Geometry: final body of the model. Coordinates: model frame, mm. Give positions to 0.01 mm unless a question says otherwise; leave off trailing zeros. Loops run counter-clockwise (first coordinate to the right, second up) from the corner with the lowest first, then second, coordinate; pieces in that order, holes last. Notation, with made-up numbers: (-39.75, 51.5) - (-23.75, 51.5) arc R17 ccw to (-23.75, 75.5) - close; hole circle Ø6 at (78, 69). An arc over 180 degrees is marked (long way). Answer in a Markdown table with one row per item.
from build123d import *

# Parameters (mm, degrees)
F0_W     = 155.681744
F0_H     = 103.419952
F1_DEPTH = 20
F2_ANGLE = -180
F3_R     = 5


with BuildPart() as f1:
    # F0 (on Top) → F1 (new body)
    with BuildSketch(Plane.XY):
        Rectangle(F0_W, F0_H)
        with BuildLine():
            ThreePointArc((0, 30.621955), (21.652992, 21.652992), (30.621955, 0))
            ThreePointArc((30.621955, 0), (21.652992, -21.652992), (0, -30.621955))
            ThreePointArc((0, -30.621955), (-30.621955, 0), (0, 30.621955))
        make_face(mode=Mode.SUBTRACT)
        with BuildLine():
            Line((0, -30.621955), (0, 30.621955))
            ThreePointArc((0, 30.621955), (-30.621955, 0), (0, -30.621955))
        make_face()
        with BuildLine():
            ThreePointArc((0, -30.621955), (21.652992, -21.652992), (30.621955, 0))
            ThreePointArc((30.621955, 0), (21.652992, 21.652992), (0, 30.621955))
            Line((0, 30.621955), (0, -30.621955))
        make_face()
    extrude(amount=-F1_DEPTH)

    # F0 (on Top) → F2 (revolve)
    with BuildSketch(Plane.XY):
        with BuildLine():
            ThreePointArc((0, -30.621955), (21.652992, -21.652992), (30.621955, 0))
            ThreePointArc((30.621955, 0), (21.652992, 21.652992), (0, 30.621955))
            Line((0, 30.621955), (0, -30.621955))
        make_face()
    revolve(axis=Axis((0, 0, 0), (0, 1, 0)), revolution_arc=F2_ANGLE)

    # F3
    f3_edges = [f1.edges().sort_by_distance(p)[0] for p in [
        (-77.840872, 0, 0),
        (0, -51.709976, 0),
        (77.840872, 0, 0),
        (0, 51.709976, 0),
    ]]
    fillet(f3_edges, radius=F3_R)


solid = f1.part
Q1. Cut plane B-B (x = -57). Output: boundary loops of the cut face in (y, z), and give its area (3 significant figures).
Check values:
| item | result |
|---|---|
| outline | (-51.71, -20) - (51.71, -20) - (51.71, -5) arc R5 ccw to (46.71, 0) - (-46.71, 0) arc R5 ccw to (-51.71, -5) - close |
| area | 2,060 mm² |
Q2. Cut plane A-A (y = -41.5). Output: boundary loops of the cut face in (x, z), and give its area (3 significant figures).
Check values:
| item | result |
|---|---|
| outline | (-77.84, -20) - (77.84, -20) - (77.84, -5) arc R5 ccw to (72.84, 0) - (-72.84, 0) arc R5 ccw to (-77.84, -5) - close |
| area | 3,100 mm² |
Q3. First-contact query: pin 1 (1 mm diameter, centred on x = -14.5, y = 6, fed in from +Z); pin 2 (5 mm diameter, centred on x = 25.5, z = 7, fed in from -Y); pin 3 (6 mm diameter, centred on x = 43, y = -8, fed in from +Z). Flat tips, straight axial feed; report the tip coordinate or a pass-through.
Check values:
| item | result |
|---|---|
| pin 1 | z = 26.59 |
| pin 2 | y = -19.09 |
| pin 3 | z = 0 |
Q4. Material intervals for line 1 along Z through (x, y) = (38.5, 42.5); line 2 along X through (y, z) = (47.5, -2); line 3 along X through (y, z) = (-1.5, 25), sorted ascending.
Check values:
| item | result |
|---|---|
| line 1 | -20 to 0 |
| line 2 | -76.84 to 76.84 |
| line 3 | -17.62 to 17.62 |
